from build123d import *

# Parameters (mm, degrees)
F0_R     = 2.54
F1_DEPTH = 7.9375


with BuildPart() as f1:
    # F0 (on Top) → F1 (new body)
    with BuildSketch(Plane.XY):
        with BuildLine():
            Line((111.125, 3.96875), (0, 3.96875))
            Line((0, 3.96875), (0, 2.54))
            ThreePointArc((0, 2.54), (1.796051, 1.796051), (2.54, 0))
            ThreePointArc((2.54, 0), (1.796051, -1.796051), (0, -2.54))
            Line((0, -2.54), (0, -3.96875))
            Line((0, -3.96875), (111.125, -3.96875))
            Line((111.125, -3.96875), (111.125, -2.54))
            ThreePointArc((111.125, -2.54), (108.585, 0), (111.125, 2.54))
            Line((111.125, 2.54), (111.125, 3.96875))
        make_face()
        with Locations((7.9375, 0)):
            Circle(F0_R, mode=Mode.SUBTRACT)
        with Locations((15.875, 0)):
            Circle(F0_R, mode=Mode.SUBTRACT)
        with Locations((23.8125, 0)):
            Circle(F0_R, mode=Mode.SUBTRACT)
        with Locations((31.75, 0)):
            Circle(F0_R, mode=Mode.SUBTRACT)
        with Locations((39.6875, 0)):
            Circle(F0_R, mode=Mode.SUBTRACT)
        with Locations((47.625, 0)):
            Circle(F0_R, mode=Mode.SUBTRACT)
        with Locations((55.5625, 0)):
            Circle(F0_R, mode=Mode.SUBTRACT)
        with Locations((63.5, 0)):
            Circle(F0_R, mode=Mode.SUBTRACT)
        with Locations((71.4375, 0)):
            Circle(F0_R, mode=Mode.SUBTRACT)
        with Locations((79.375, 0)):
            Circle(F0_R, mode=Mode.SUBTRACT)
        with Locations((87.3125, 0)):
            Circle(F0_R, mode=Mode.SUBTRACT)
        with Locations((95.25, 0)):
            Circle(F0_R, mode=Mode.SUBTRACT)
        with Locations((103.1875, 0)):
            Circle(F0_R, mode=Mode.SUBTRACT)
        with BuildLine():
            Line((0, 2.54), (0, 3.96875))
            ThreePointArc((0, 3.96875), (-3.96875, 0), (0, -3.96875))
            Line((0, -3.96875), (0, -2.54))
            ThreePointArc((0, -2.54), (-2.54, 0), (0, 2.54))
        make_face()
        with BuildLine():
            ThreePointArc((111.125, -3.96875), (115.09375, 0), (111.125, 3.96875))
            Line((111.125, 3.96875), (111.125, 2.54))
            ThreePointArc((111.125, 2.54), (112.921051, 1.796051), (113.665, 0))
            ThreePointArc((113.665, 0), (112.921051, -1.796051), (111.125, -2.54))
            Line((111.125, -2.54), (111.125, -3.96875))
        make_face()
    extrude(amount=F1_DEPTH)


solid = f1.part
Work out the finished part from the listing and answer in its coordinate system (mm). Round coordinates to 2 decimals unless told otherwise and drop trailing zeros. Write each loop counter-clockwise with the first axis right and the second up, starting at its lowest first coordinate (ties: lowest second). Pieces come first, ordered by that corner, then holes. Notation, with made-up numbers: (-38, 11) -> (-14, 11) arc R14 cw to (-14, 35) -> close; hole circle Ø9 at (-15.5, 26). An arc over 180 degrees is marked (long way). Write each question's results on one line, items separated by ' | '.
Item 1: The mould has two halves that part along Y. Classify faces 1 (the face through (55, 3, 7.938)), 2 (the face through (55, -3.969, 4)), 3 (the face through (69.422, -1.546, 3.913)), 4 (the face through (65.846, -0.973, 3.913)): +Y half, -Y half, draft (parallel to the pull), parting line (faces both ways), or undercut.
Result set:
face 1: draft | face 2: -Y half | face 3: undercut | face 4: undercut
Item 2: A cutting plane is placed at C-C, the plane x = 14.5. Determine the outline of the cut face in (y, z).
Result set:
outline: (-3.97, 0) -> (-2.14, 0) -> (-2.14, 7.94) -> (-3.97, 7.94) -> close; (2.14, 0) -> (3.97, 0) -> (3.97, 7.94) -> (2.14, 7.94) -> close
Item 3: Find the intervals of material crossed by line 1 along Y through (x, z) = (31.75, 3.5); line 2 along Y through (x, z) = (49.5, 2.75), in increasing order. Write a range as [from, to].
Result set:
line 1: [-3.97, -2.54], [2.54, 3.97] | line 2: [-3.97, -1.71], [1.71, 3.97]
Item 4: A flat-ended cylindrical pin translates along its axis: P1, Ø3, axis at y = 2.5, z = 3, coming from the +X side. Find the tip coordinate at first contact, or state that the pin passes through.
Result set:
P1: x = 114.97
Item 5: A cutting plane is placed at A-A, the plane x = 63.5. Determine the outline of the cut face in (y, z), plus the area to 3 significant figures.
Result set:
outline: (-3.97, 0) -> (-2.54, 0) -> (-2.54, 7.94) -> (-3.97, 7.94) -> close; (2.54, 0) -> (3.97, 0) -> (3.97, 7.94) -> (2.54, 7.94) -> close | area: 22.7 mm^2
Item 6: A cutting plane is placed at B-B, the plane z = 5. Count the separate pieces of the cut face and the enclosed holes in it, plus the area to 3 significant figures.
Result set:
separate pieces: 1 | enclosed holes: 15 | area: 628 mm^2
